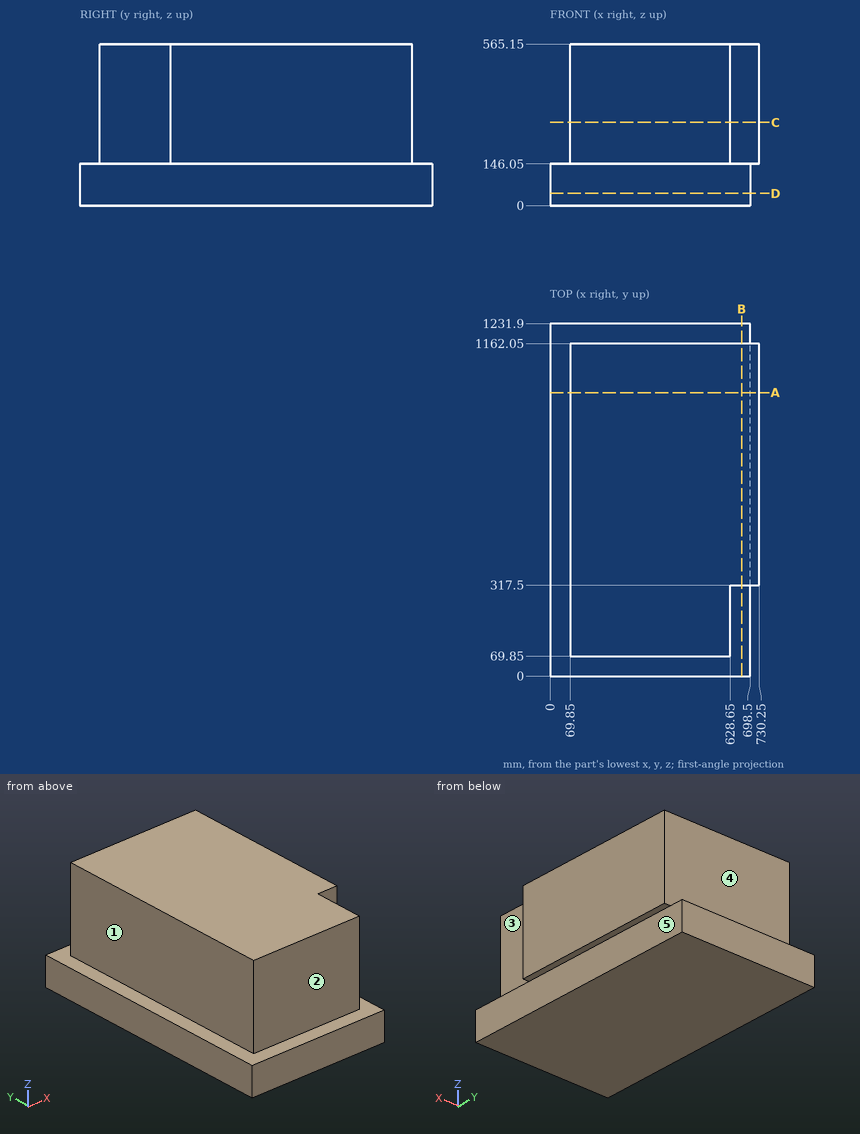
Part print with two shaded views. Sizes in mm from the minimum x, y, z corner. A direction names the side the tool comes from. Give positions to 0.01 mm unless a question says otherwise; leave off trailing zeros. Order: outer loops, then holes, each group sorted by start corner. A loop starts at its lowest first (then second) coordinate and runs counter-clockwise, first axis right, second up. Notation, with made-up numbers: (28.5, 78.5) - (55.5, 78.5) arc R15 cw to (55.5, 89.5) - close; hole circle Ø3 at (56, 10). An arc over 180 degrees is marked (long way). Write each question's results on one line, items separated by ' | '.
1. Pin check, flat tips, straight feed: pin 1 (5 mm diameter, centred on x = 187.5, z = 390.5, fed in from +Y); pin 2 (5 mm diameter, centred on x = 656.5, y = 249.5, fed in from -Z); pin 3 (16 mm diameter, centred on x = 709, y = 697, fed in from -Z); pin 4 (6 mm diameter, centred on y = 692, z = 202.5, fed in from -X). Stop position of each tip, or through.
Calculated:
pin 1: stops at y = 1162.05 | pin 2: stops at z = 0 | pin 3: stops at z = 146.05 | pin 4: stops at x = 69.85
2. Saw through at C-C on z = 291. List the corners of the cut face in (x, y), and give its area (3 significant figures).
Calculated:
outline: (69.85, 69.85) - (628.65, 69.85) - (628.65, 317.5) - (730.25, 317.5) - (730.25, 1162.05) - (69.85, 1162.05) - close | area: 696,000 mm2
3. Saw through at A-A on y = 991. List the corners of the cut face in (x, z).
Calculated:
outline: (0, 0) - (698.5, 0) - (698.5, 146.05) - (730.25, 146.05) - (730.25, 565.15) - (69.85, 565.15) - (69.85, 146.05) - (0, 146.05) - close
4. Saw through at B-B on x = 669. List the corners of the cut face in (y, z).
Calculated:
outline: (0, 0) - (1231.9, 0) - (1231.9, 146.05) - (1162.05, 146.05) - (1162.05, 565.15) - (317.5, 565.15) - (317.5, 146.05) - (0, 146.05) - close
5. 3-axis set-ups, long thin cutter, end or side, ignore diameter. For the marked faces 1, 2, 3, 4 and 5: which of +Z, -Z, +X, -X, +Y, -Y reach the whole face in a straight line?
Calculated:
face 1: +Z, -X, +Y, -Y | face 2: +Z, +X, -X, -Y | face 3: +Z, +X, -Y | face 4: +Z, +X, -X, +Y | face 5: -Z, +X, +Y, -Y
6. Saw through at D-D on z = 42.5. List the corners of the cut face in (x, y).
Calculated:
outline: (0, 0) - (698.5, 0) - (698.5, 1231.9) - (0, 1231.9) - close
7. Probe L1, parallel to X at y = 240, z = 472.5; L2, parallel to Y at x = 379.5, z = 279; L3, parallel to Z at x = 671, y = 97. List the from-to ranges inside material, lowest first. Write a range as from..to.
Calculated:
L1: x = 69.85..628.65 | L2: y = 69.85..1162.05 | L3: z = 0..146.05
